from build123d import *

# Parameters (mm, degrees)
SKETCH1_R                = 15
BOSS_EXTRUDE1_DEPTH      = 20
FILLET1_R                = 10
BOSS_EXTRUDE2_DEPTH      = 300
BOSS_EXTRUDE2_DEPTH_BACK = 300
SKETCH2_W                = 20
SKETCH2_H                = 20
SKETCH3_W                = 403
SKETCH3_H                = 20
BOSS_EXTRUDE3_DEPTH      = 23
BOSS_EXTRUDE4_DEPTH      = 50
SKETCH5_R                = 2.5
SKETCH5_R_2              = 5
BOSS_EXTRUDE5_DEPTH      = 10


with BuildPart() as part:
    # Sketch1 → Boss-Extrude1 (new body)
    with BuildSketch(Plane(origin=(0, 0, 0), x_dir=(0, 0, -1), z_dir=(1, 0, 0))):
        with BuildLine():
            Line((-277.087121525, 516.456439237), (-32.912878475, 516.456439237))
            ThreePointArc((-32.912878475, 516.456439237), (7.67766953, 524.134108767), (0, 483.543560763))
            Line((0, 483.543560763), (0, -483.543560763))
            Line((0, -483.543560763), (-500, -483.543560763))
            Line((-500, -483.543560763), (-315.275252317, -277.015014289))
            ThreePointArc((-315.275252317, -277.015014289), (-275.879773408, -247.969529867), (-300.368132467, -290.348347623))
            Line((-300.368132467, -290.348347623), (-455.27864045, -463.543560763))
            Line((-455.27864045, -463.543560763), (-20, -463.543560763))
            Line((-20, -463.543560763), (-20, 483.543560763))
            ThreePointArc((-20, 483.543560763), (-27.67766953, 488.778769708), (-32.912878475, 496.456439237))
            Line((-32.912878475, 496.456439237), (-277.087121525, 496.456439237))
            ThreePointArc((-277.087121525, 496.456439237), (-325, 506.456439237), (-277.087121525, 516.456439237))
        make_face()
        with Locations((-292.546440075, -266.603429679)):
            Circle(SKETCH1_R, mode=Mode.SUBTRACT)
        with Locations((-300, 506.456439237)):
            Circle(SKETCH1_R, mode=Mode.SUBTRACT)
        with Locations((-10, 506.456439237)):
            Circle(SKETCH1_R, mode=Mode.SUBTRACT)
    extrude(amount=BOSS_EXTRUDE1_DEPTH)

    # Fillet1
    fillet1_edges = [part.edges().sort_by_distance(p)[0] for p in [
        (10, -483.543560763, 500),
    ]]
    fillet(fillet1_edges, radius=FILLET1_R)


with BuildPart() as body_2:
    # Mirror2: mirrored copy
    add(part.part.mirror(Plane(origin=(-115, 0, 0), x_dir=(0, 0, 1), z_dir=(1, 0, 0))))


with BuildPart() as part_1:
    add(part.part)

    add(body_2.part)  # Boss-Extrude2 merges body 2
    # Sketch2 → Boss-Extrude2 (add, two sides: drawn at the far end of the back side and taken through both)
    with BuildSketch(Plane(origin=(-115, 0, 0), x_dir=(0, 0, -1), z_dir=(1, 0, 0)).offset(-BOSS_EXTRUDE2_DEPTH_BACK)):
        with Locations((-10, -473.543560763)):
            Rectangle(SKETCH2_W, SKETCH2_H)
    extrude(amount=BOSS_EXTRUDE2_DEPTH + BOSS_EXTRUDE2_DEPTH_BACK)

    # Sketch3 → Boss-Extrude3 (add)
    with BuildSketch(Plane(origin=(20, 0, 0), x_dir=(0, 0, -1), z_dir=(1, 0, 0))):
        with Locations((-201.5, 319.456439237)):
            Rectangle(SKETCH3_W, SKETCH3_H)
    extrude(amount=-BOSS_EXTRUDE3_DEPTH)

    # Sketch4 → Boss-Extrude4 (add)
    with BuildSketch(Plane.ZY.offset(250)):
        Polygon((330, -293.477782675), (315.09288015, -306.811116008), (321.759546817, -314.264675933), (336.666666667, -300.9313426), align=None)
    extrude(amount=BOSS_EXTRUDE4_DEPTH)

    # Sketch5 → Boss-Extrude5 (add)
    with BuildSketch(Plane.ZY.offset(300)):
        with BuildLine():
            Line((317.152993446, -318.384902525), (345.480143996, -293.048328829))
            ThreePointArc((345.480143996, -293.048328829), (348.692480121, -287.145673106), (347.443414331, -280.542622098))
            Line((347.443414331, -280.542622098), (320.125662167, -233.879195794))
            ThreePointArc((320.125662167, -233.879195794), (316.469583424, -230.256048136), (311.495725166, -228.9313426))
            Line((311.495725166, -228.9313426), (267.229084741, -228.9313426))
            ThreePointArc((267.229084741, -228.9313426), (260.158016929, -231.860274788), (257.229084741, -238.9313426))
            Line((257.229084741, -238.9313426), (257.229084741, -310.9313426))
            ThreePointArc((257.229084741, -310.9313426), (260.158016929, -318.002410412), (267.229084741, -320.9313426))
            Line((267.229084741, -320.9313426), (310.486326779, -320.9313426))
            ThreePointArc((310.486326779, -320.9313426), (314.054547677, -320.27306619), (317.152993446, -318.384902525))
        make_face()
        with Locations((317.547753068, -280.286250567)):
            Circle(SKETCH5_R, mode=Mode.SUBTRACT)
        with Locations((268.196113094, -281.413791415)):
            Circle(SKETCH5_R, mode=Mode.SUBTRACT)
        with Locations((291.895454063, -238.110247055)):
            Circle(SKETCH5_R, mode=Mode.SUBTRACT)
        with Locations((292.546440075, -266.603429679)):
            Circle(SKETCH5_R_2, mode=Mode.SUBTRACT)
    extrude(amount=BOSS_EXTRUDE5_DEPTH)


solid = part_1.part
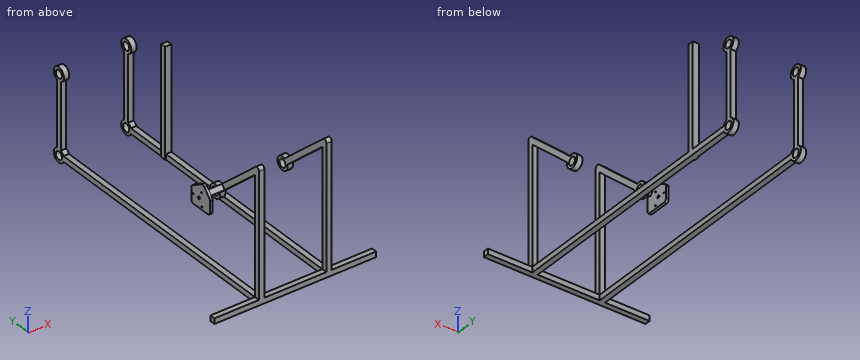
Could you check a few things on this model? Use its own coordinates, in mm. Coordinates: 2 decimals unless noted, no trailing zeros. Order: outer loops, then holes, each group sorted by start corner. A loop starts at its lowest first (then second) coordinate and runs counter-clockwise, first axis right, second up.
Q1. Please list where these lines run through material, in increasing order: L1, parallel to Y at x = 6.75, z = 10; L2, parallel to Y at x = 6, z = 300; L3, parallel to Z at x = -234, y = -321.
Q2. Suppose I cut it at A-A on x = -262. Please give me the cut outline in (y, z), and give its area (3 significant figures).
Q3. Will this pin go through, and if not, where does the flat tip stop? pin 1 (5 mm diameter, centred on x = -304, y = -266, fed in from -Z).
Q4. Suppose I cut it at B-B on z = 229. Please give me the cut outline in (x, y), and give its area (3 significant figures).
Q5. Suppose I cut it at C-C on y = 213. Please give me the cut outline in (x, z), and give its area (3 significant figures).
Q6. Suppose I cut it at D-D on z = 423. Please give me the cut outline in (x, y), and give its area (3 significant figures).
Answer:
1. L1: y = -483.54 to 491.46, 521.46 to 531.46
1. L2: y = -483.54 to -463.54, -290.47 to -279.62, -253.59 to -242.74, 309.46 to 329.46, 481.46 to 491.46, 521.46 to 531.46
1. L3: z = 0 to 20, 327.78 to 354.62
2. outline: (-483.54, 0) - (-463.54, 0) - (-463.54, 20) - (-483.54, 20) - close; (-314.26, 321.76) - (-306.81, 315.09) - (-293.48, 330) - (-300.93, 336.67) - close
2. area: 600 mm2
3. pin 1: stops at z = 257.23
4. outline: (-250, -483.54) - (-230, -483.54) - (-230, -463.54) - (-250, -463.54) - close; (-250, 496.46) - (-230, 496.46) - (-230, 516.46) - (-250, 516.46) - close; (-3, 309.46) - (20, 309.46) - (20, 329.46) - (-3, 329.46) - close; (0, -483.54) - (20, -483.54) - (20, -463.54) - (0, -463.54) - close; (0, 496.46) - (20, 496.46) - (20, 516.46) - (0, 516.46) - close
4. area: 2,060 mm2
5. outline: (-250, 0) - (-230, 0) - (-230, 20) - (-250, 20) - close; (0, 0) - (20, 0) - (20, 20) - (0, 20) - close
5. area: 800 mm2
6. outline: (-250, -483.54) - (-230, -483.54) - (-230, -463.54) - (-250, -463.54) - close; (-250, -427.45) - (-230, -427.45) - (-230, -397.45) - (-250, -397.45) - close; (0, -483.54) - (20, -483.54) - (20, -463.54) - (0, -463.54) - close; (0, -427.45) - (20, -427.45) - (20, -397.45) - (0, -397.45) - close
6. area: 2,000 mm2
